from build123d import *

# Parameters (mm, degrees)
SKETCH1_R               = 11
BOSS_EXTRUDE1_DEPTH     = 3.5
CUT_EXTRUDE3_REACH      = 46.858
CUT_EXTRUDE3_END_RADIUS = 13
SKETCH2_W               = 3
SKETCH2_H               = 8
CIRPATTERN1_COUNT       = 8


with BuildPart() as part:
    # Sketch1 → Boss-Extrude1 (new, symmetric)
    with BuildSketch(Plane.XY):
        Polygon((8.284271247, 20), (-8.284271247, 20), (-20, 8.284271247), (-20, -8.284271247), (-8.284271247, -20), (8.284271247, -20), (20, -8.284271247), (20, 8.284271247), align=None)
        Circle(SKETCH1_R, mode=Mode.SUBTRACT)
    extrude(amount=BOSS_EXTRUDE1_DEPTH, both=True)

    # Cut-Extrude3: up to this cylinder (the profile starts outside it)
    cut_extrude3_end = Plane(origin=(0, 0, 0), z_dir=(0, 0, -1)) * Cylinder(CUT_EXTRUDE3_END_RADIUS, 120.716, mode=Mode.PRIVATE)
    # Sketch2 → Cut-Extrude3 (cut, up to the surface)
    with BuildSketch(Plane(origin=(0, -20, 0), x_dir=(-1, 0, 0), z_dir=(0, -1, 0)), mode=Mode.PRIVATE) as cut_extrude3_sk1:
        Rectangle(SKETCH2_W, SKETCH2_H)
    cut_extrude3_tool1 = extrude(cut_extrude3_sk1.sketch, amount=-CUT_EXTRUDE3_REACH, mode=Mode.PRIVATE) - cut_extrude3_end
    cut_extrude3 = cut_extrude3_tool1.solids().sort_by_distance((0, -20, 0))[0]
    add(cut_extrude3, mode=Mode.SUBTRACT)

    # CirPattern1: Cut-Extrude3 ×8 about axis
    cirpattern1_axis = Axis((0, 0, 0), (0, 0, 1))
    for i in range(1, CIRPATTERN1_COUNT):
        add(cut_extrude3.rotate(cirpattern1_axis, i * 360 / CIRPATTERN1_COUNT), mode=Mode.SUBTRACT)


solid = part.part
Input: part model. Units: mm. Frame: model coordinates. A direction names the side the tool comes from. Coordinates: 2 decimals unless noted, no trailing zeros. Loops run counter-clockwise (first coordinate to the right, second up) from the corner with the lowest first, then second, coordinate; pieces in that order, holes last. Notation, with made-up numbers: (21, 76) -> (35, 76) arc R34 ccw to (35, 112) -> close; hole circle Ø5 at (21.25, -13.5). An arc over 180 degrees is marked (long way). One line per item, written item: value.
(1) Set-up query: faces 1 (the face through (-17, 1.5, 0)), 2 (the face through (1.5, 17, 0)), 3 (the face through (-9.207, 9.177, -0.049)), 4 (the face through (-10.716, -17.568, 0.049)), 5 (the face through (17, 1.5, 0)). Return all of +Z, -Z, +X, -X, +Y, -Y with unobstructed straight access to the full face (end or side cutting, diameter ignored); none if empty.
Answer below:
face 1: +Z, -Z, -X
face 2: +Z, -Z, +Y
face 3: +Z, -Z
face 4: +Z, -Z, -X, -Y
face 5: +Z, -Z, +X
(2) Cut plane C-C (y = -11.5). Output: boundary loops of the cut face in (x, z).
Answer below:
outline: (-16.78, -3.5) -> (-13.62, -3.5) -> (-13.62, 3.5) -> (-16.78, 3.5) -> close; (-9.38, -3.5) -> (9.38, -3.5) -> (9.38, 3.5) -> (-9.38, 3.5) -> close; (13.62, -3.5) -> (16.78, -3.5) -> (16.78, 3.5) -> (13.62, 3.5) -> close
(3) Ray query, line 1 along X through (y, z) = (-11.5, 0.5); line 2 along X through (y, z) = (10, -2.5); line 3 along X through (y, z) = (4, 2). Return the intervals inside material, ascending.
Answer below:
line 1: x = -16.78 to -13.62, -9.38 to 9.38, 13.62 to 16.78
line 2: x = -18.28 to -12.12, -8.31 to -4.58, 4.58 to 8.31, 12.12 to 18.28
line 3: x = -20 to -10.25, 10.25 to 20
(4) Draft query along X for faces 6 (the face through (-13, 0, 0)), 7 (the face through (-5, -20, 0)), 8 (the face through (-12.73, -10.61, 0.05)). Return one class per face: pulls with the +X half, pulls with the -X half, needs draft (parallel to the pull), parting line crosses it, or undercut.
Answer below:
face 6: pulls with the -X half
face 7: needs draft
face 8: undercut
(5) Pin query (flat end, axial travel): pin 1 Ø3.5 at (y, z) = (15, 1) entering from +X; pin 2 Ø2 at (y, z) = (-18, -1.5) entering from -X; pin 3 Ø12 at (x, y) = (-0.5, -3.5) entering from +Z; pin 4 Ø10 at (x, y) = (6.5, -6.5) entering from +Z. Return the tip coordinate at first contact, or that it passes through.
Answer below:
pin 1: stops at x = 13.08
pin 2: stops at x = -11.28
pin 3: passes through
pin 4: stops at z = 3.5
(6) Cut plane A-A (x = 0). Output: boundary loops of the cut face in (y, z), then the cut area to 3 significant figures.
Answer below:
outline: (-13, -3.5) -> (-11, -3.5) -> (-11, 3.5) -> (-13, 3.5) -> close; (11, -3.5) -> (13, -3.5) -> (13, 3.5) -> (11, 3.5) -> close
area: 28.0 mm2
